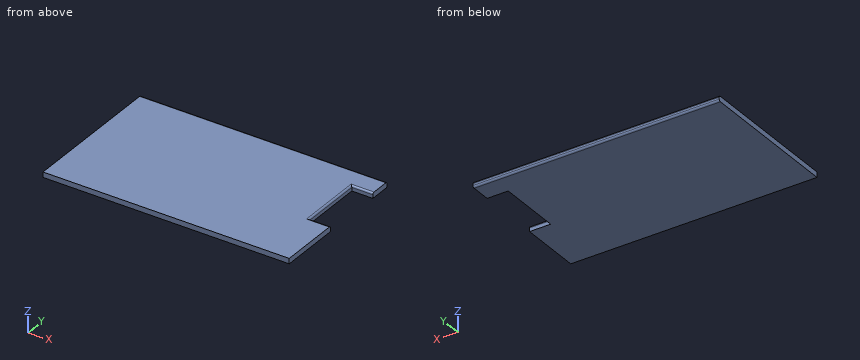
from build123d import *

# Parameters (mm, degrees)
F1_DEPTH = 19.05
F2_R     = 6.35


with BuildPart() as f1:
    # F0 (on Top) → F1 (new body)
    with BuildSketch(Plane.XY):
        Polygon((-444.5, -263.525), (444.5, -263.525), (444.5, -41.275), (368.3, -41.275), (368.3, 187.325), (444.5, 187.325), (444.5, 263.525), (-444.5, 263.525), align=None)
    extrude(amount=F1_DEPTH)

    # F2
    f2_edges = [f1.edges().sort_by_distance(p)[0] for p in [
        (0, 263.525, 19.05),
        (0, 263.525, 0),
        (406.4, -41.275, 19.05),
        (368.3, 73.025, 19.05),
        (406.4, 187.325, 19.05),
    ]]
    fillet(f2_edges, radius=F2_R)


solid = f1.part
Model file for the job. Use its own axes, mm. Round coordinates to 2 decimals unless told otherwise and drop trailing zeros. Loops run counter-clockwise (first coordinate to the right, second up) from the corner with the lowest first, then second, coordinate; pieces in that order, holes last. Notation, with made-up numbers: (24.25, 54) - (45.25, 54) arc R34 ccw to (45.25, 87) - close; hole circle Ø1 at (22, 37). An arc over 180 degrees is marked (long way). Write each question's results on one line, items separated by ' | '.
(1) Pin check, flat tips, straight feed: pin 1 (6.5 mm diameter, centred on y = 17, z = 6.5, fed in from +X); pin 2 (1.5 mm diameter, centred on x = -45, z = 3, fed in from +Y). Stop position of each tip, or through.
Answer below:
pin 1: stops at x = 368.3 | pin 2: stops at y = 262.97
(2) Wall check: L1, parallel to Y at x = 408, z = 12.5 (3 decimals); L2, parallel to X at y = 110, z = 7; L3, parallel to Y at x = 376.5, z = 18.25 (3 decimals). Give the ranges that are in metal, low to high.
Answer below:
L1: y = -263.525 to -41.275, 187.325 to 263.525 | L2: x = -444.5 to 368.3 | L3: y = -263.525 to -44.54, 190.59 to 260.26
(3) Saw through at A-A, the plane y = -31. List the corners of the cut face in (x, z).
Answer below:
outline: (-444.5, 0) - (368.3, 0) - (368.3, 12.7) arc R6.35 ccw to (361.95, 19.05) - (-444.5, 19.05) - close
